Input: dimensioned drawing with shaded views. Units: mm. Origin: part minimum x, y, z. A direction names the side the tool comes from. Give positions to 0.01 mm unless a question says otherwise; leave off trailing zeros. Loops run counter-clockwise (first coordinate to the right, second up) from the corner with the lowest first, then second, coordinate; pieces in that order, holes last.
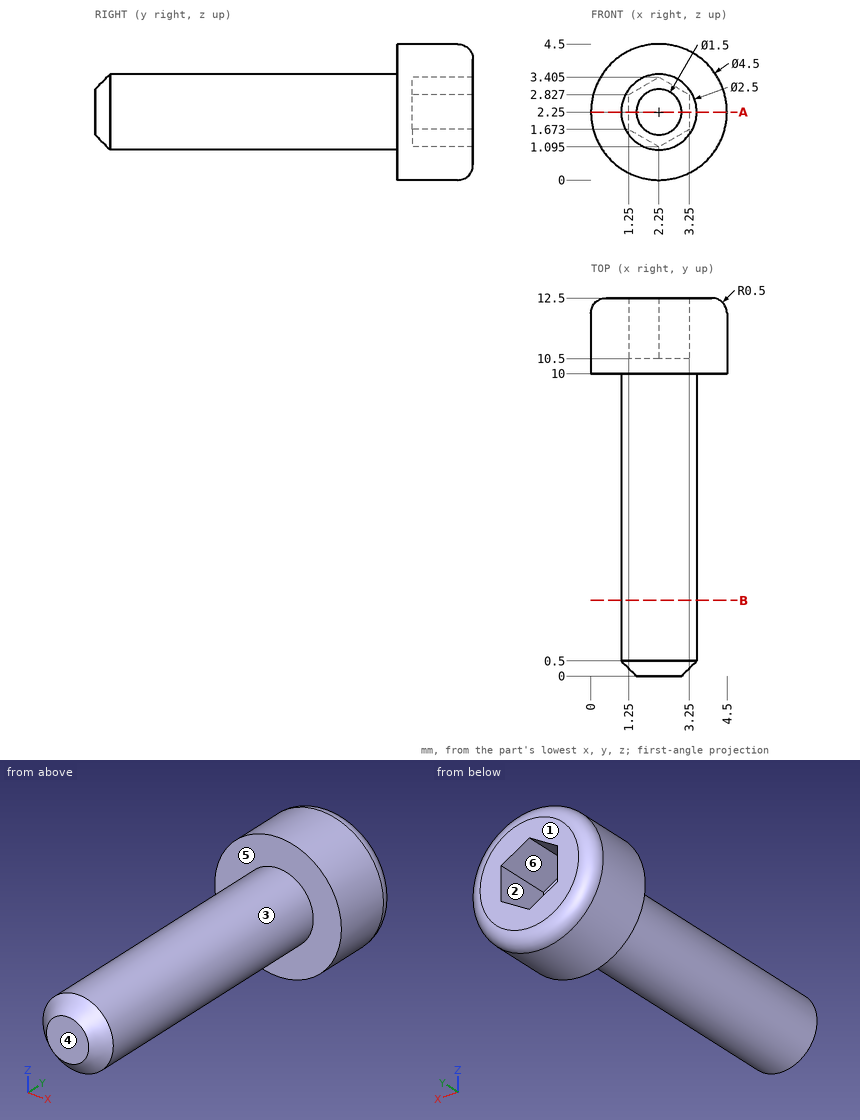
(1) Section B-B, the plane y = 2.5. Return the cut outline in (x, z).
A:
outline: circle Ø2.5 at (2.25, 2.25)
(2) Mould query, pull axis Z, two halves, no side actions, for the marked faces 1, 2 and 3. Classes: pulls with the +Z half, pulls with the -Z half, needs draft (parallel to the pull), parting line crosses it, or undercut.
A:
face 1: needs draft
face 2: undercut
face 3: parting line crosses it
(3) Section A-A, the plane z = 2.25. Return the cut outline in (x, y), then the cut area to 3 significant figures.
A:
outline: (0, 10) - (1, 10) - (1, 0.5) - (1.5, 0) - (3, 0) - (3.5, 0.5) - (3.5, 10) - (4.5, 10) - (4.5, 12) arc R0.5 ccw to (4, 12.5) - (3.25, 12.5) - (3.25, 10.5) - (1.25, 10.5) - (1.25, 12.5) - (0.5, 12.5) arc R0.5 ccw to (0, 12) - close
area: 31.9 mm2
(4) Reachability of the marked faces 4, 5 and 6 from +Z, -Z, +X, -X, +Y, -Y: full face, straight path, thin tool, end or side. Return the list, or none.
A:
face 4: +Z, -Z, +X, -X, -Y
face 5: -Y
face 6: +Y
(5) First-contact query: pin 1 (0.6 mm diameter, centred on x = 2.5, z = 2.5, fed in from +Y); pin 2 (1.5 mm diameter, centred on x = 3.5, y = 6, fed in from -Z) (1 decimal). Flat tips, straight axial feed; report the tip coordinate or a pass-through.
A:
pin 1: stops at y = 10.5
pin 2: stops at z = 1.1
(6) Ray query, line 1 along Y through (x, z) = (2.5, 0.8); line 2 along Z through (x, y) = (2.2, 9.5); line 3 along X through (y, z) = (8, 1.5). Return the intervals inside material, ascending.
A:
line 1: y = 10 to 12.5
line 2: z = 1 to 3.5
line 3: x = 1.25 to 3.25
